```python
from build123d import *

# Parameters (mm, degrees)
SKETCH1_W               = 30
SKETCH1_H               = 18
BOSS_EXTRUDE1_DEPTH     = 1.5
SKETCH2_W               = 9.352993505
SKETCH2_H               = 9.546694554
BOSS_EXTRUDE2_DEPTH     = 3
SKETCH3_R               = 0.926140641
CUT_EXTRUDE1_DEPTH      = 2.5
CIRPATTERN1_COUNT       = 2
MIRROR1_COPY_1_SKETCH_R = 0.926140641
MIRROR1_COPY_1_DEPTH    = 2.5


with BuildPart() as part:
    # Sketch1 → Boss-Extrude1 (new body)
    with BuildSketch(Plane(origin=(0, 0, 0), x_dir=(1, 0, 0), z_dir=(0, 1, 0))):
        Rectangle(SKETCH1_W, SKETCH1_H)
    extrude(amount=BOSS_EXTRUDE1_DEPTH)

    # Sketch2 → Boss-Extrude2 (add)
    with BuildSketch(Plane(origin=(0, 1.5, 0), x_dir=(1, 0, 0), z_dir=(0, 1, 0))):
        with Locations((1.252138924, -3.867103084)):
            Rectangle(SKETCH2_W, SKETCH2_H)
    extrude(amount=BOSS_EXTRUDE2_DEPTH)

    # Sketch3 → Cut-Extrude1 (cut, through all)
    with BuildSketch(Plane(origin=(0, 1.5, 0), x_dir=(1, 0, 0), z_dir=(0, 1, 0))):
        with Locations((-13.228024261, 7.468220339)):
            Circle(SKETCH3_R)
        with Locations((-13.228024261, 4.702212806)):
            Circle(SKETCH3_R)
    cut_extrude1 = extrude(amount=-CUT_EXTRUDE1_DEPTH, mode=Mode.SUBTRACT)

    # CirPattern1: Cut-Extrude1 ×2 about axis
    cirpattern1_axis = Axis((0, 0, 0), (0, 1, 0))
    for i in range(1, CIRPATTERN1_COUNT):
        add(cut_extrude1.rotate(cirpattern1_axis, i * 360 / CIRPATTERN1_COUNT), mode=Mode.SUBTRACT)

    # Mirror1: Cut-Extrude1 across plane
    add(cut_extrude1.mirror(Plane(origin=(0, 0, 0), x_dir=(0, 0, 1), z_dir=(1, 0, 0))), mode=Mode.SUBTRACT)

    # Mirror1 copy 1 sketch → Mirror1 copy 1 (cut, through all)
    with BuildSketch(Plane(origin=(0, 1.5, 0), x_dir=(1, 0, 0), z_dir=(0, 1, 0))):
        with Locations((-13.228024261, -7.468220339)):
            Circle(MIRROR1_COPY_1_SKETCH_R)
        with Locations((-13.228024261, -4.702212806)):
            Circle(MIRROR1_COPY_1_SKETCH_R)
    extrude(amount=-MIRROR1_COPY_1_DEPTH, mode=Mode.SUBTRACT)


solid = part.part
```
The model under review builds one solid part; all positions refer to its coordinate system, in mm. A direction names the side the tool comes from. Give positions to 0.01 mm unless a question says otherwise; leave off trailing zeros. Write each loop counter-clockwise with the first axis right and the second up, starting at its lowest first coordinate (ties: lowest second). Pieces come first, ordered by that corner, then holes. Notation, with made-up numbers: (79.5, 83) -> (119.5, 83) arc R12 cw to (119.5, 101) -> close; hole circle Ø7 at (59, 58.25). An arc over 180 degrees is marked (long way). Answer in a Markdown table with one row per item.
1) Add section D-D on z = 2. State the section outline as (x, y) points.
Worked answers:
| item | result |
|---|---|
| outline | (-15, 0) -> (15, 0) -> (15, 1.5) -> (5.93, 1.5) -> (5.93, 4.5) -> (-3.42, 4.5) -> (-3.42, 1.5) -> (-15, 1.5) -> close |
2) Tool access review of faces 4 (the flat face through (5.929, 3, 4)), 5 (the flat face through (-3.424, 3, 4)), 6 (the flat face through (1, 3, 8.64)): name each direction out of +Z, -Z, +X, -X, +Y, -Y from which nothing blocks a thin tool from reaching the whole face with its end or side.
Worked answers:
| item | result |
|---|---|
| face 4 | +Z, -Z, +X, +Y |
| face 5 | +Z, -Z, -X, +Y |
| face 6 | +Z, +X, -X, +Y |
3) Add section A-A on z = -5. State the section outline as (x, y) points, plus the area to 3 significant figures.
Worked answers:
| item | result |
|---|---|
| outline | (-15, 0) -> (-14.1, 0) -> (-14.1, 1.5) -> (-15, 1.5) -> close; (-12.35, 0) -> (12.35, 0) -> (12.35, 1.5) -> (-12.35, 1.5) -> close; (14.1, 0) -> (15, 0) -> (15, 1.5) -> (14.1, 1.5) -> close |
| area | 39.7 mm² |
4) Add section C-C on y = 0.3. Count the separate pieces of the cut face and the enclosed holes in it, plus the area to 3 significant figures.
Worked answers:
| item | result |
|---|---|
| separate pieces | 1 |
| enclosed holes | 8 |
| area | 518 mm² |
5) Clearance check with flat-ended pins moving along their axes: P1, Ø1.5, axis at x = -13.23, z = -7.47, coming from the -Y side; P2, Ø2.5, axis at x = 3, y = 3, coming from the -Z side; P3, Ø2.5, axis at x = 13.23, z = 4.7, coming from the +Y side; P4, Ø2, axis at y = 3.5, z = 4, coming from the -X side. State where each tip first meets the part, or that it passes through.
Worked answers:
| item | result |
|---|---|
| P1 | through |
| P2 | z = -0.91 |
| P3 | y = 1.5 |
| P4 | x = -3.42 |
6) Add section B-B on x = -1.5. State the section outline as (y, z) points.
Worked answers:
| item | result |
|---|---|
| outline | (0, -9) -> (1.5, -9) -> (1.5, -0.91) -> (4.5, -0.91) -> (4.5, 8.64) -> (1.5, 8.64) -> (1.5, 9) -> (0, 9) -> close |
7) Mouldability with a two-part tool opening along Z and no side actions: class faces 1 (the flat face through (1, 3, -0.906)), 2 (the cylindrical face through (-12.73, 0.76, 6.687)), 3 (the flat face through (-15, 1, 0)) as +Z half, -Z half, draft (parallel to the pull), parting line (faces both ways), or undercut.
Worked answers:
| item | result |
|---|---|
| face 1 | -Z half |
| face 2 | undercut |
| face 3 | draft |
8) For L1, parallel to X at y = 0.9, z = 4.75; L2, parallel to X at y = 0.95, z = 4.25; L3, parallel to Z at x = -3, y = 2.7, list the stretches that pass through material, from the lowest coordinate up. Write a range as [from, to].
Worked answers:
| item | result |
|---|---|
| L1 | [-15, -14.15], [-12.3, 12.3], [14.15, 15] |
| L2 | [-15, -14.04], [-12.42, 12.42], [14.04, 15] |
| L3 | [-0.91, 8.64] |
